Verification items for the finished model (mm, model axes). A direction names the side the tool comes from. Coordinates: 2 decimals unless noted, no trailing zeros. Write each loop counter-clockwise with the first axis right and the second up, starting at its lowest first coordinate (ties: lowest second). Pieces come first, ordered by that corner, then holes. Notation, with made-up numbers: (-20, 41.25) -> (25, 41.25) arc R23 cw to (25, 67.25) -> close; hole circle Ø4 at (37.25, -20). An arc over 180 degrees is marked (long way). Answer in a Markdown table with one row per item.
```python
from build123d import *

# Parameters (mm, degrees)
SKETCH1_W           = 15
SKETCH1_H           = 40
BOSS_EXTRUDE2_DEPTH = 3
SKETCH2_W           = 15
SKETCH2_H           = 15
BOSS_EXTRUDE5_DEPTH = 5
CUT_EXTRUDE9_DEPTH  = 15
SKETCH14_W          = 11
SKETCH14_H          = 0.5
CUT_EXTRUDE10_DEPTH = 5
BOSS_EXTRUDE9_DEPTH = 2
SKETCH18_R          = 1.5
CUT_EXTRUDE11_DEPTH = 10


with BuildPart() as part:
    # Sketch1 → Boss-Extrude2 (new body)
    with BuildSketch(Plane.XY):
        with Locations((0.416666667, -8.072916667)):
            Rectangle(SKETCH1_W, SKETCH1_H)
    extrude(amount=BOSS_EXTRUDE2_DEPTH)

    # Sketch2 → Boss-Extrude5 (add)
    with BuildSketch(Plane(origin=(0, 0, 0), x_dir=(-1, 0, 0), z_dir=(0, 0, -1))):
        with Locations((-0.416666667, 4.427083333)):
            Rectangle(SKETCH2_W, SKETCH2_H)
    extrude(amount=BOSS_EXTRUDE5_DEPTH)

    # Sketch12 → Cut-Extrude9 (cut)
    with BuildSketch(Plane.ZY.offset(7.083333333)):
        Polygon((-5, 11.927083333), (-5, 4.427083333), (0, 11.927083333), align=None)
    extrude(amount=-CUT_EXTRUDE9_DEPTH, mode=Mode.SUBTRACT)

    # Sketch14 → Cut-Extrude10 (cut)
    with BuildSketch(Plane(origin=(0, 3.669871795, -5.504807692), x_dir=(-1, 0, 0), z_dir=(0, 0.5547001962252293, -0.8320502943378436))):
        with Locations((-0.416666667, 3.160055009)):
            Rectangle(SKETCH14_W, SKETCH14_H)
        with Locations((-0.416666667, 4.160055009)):
            Rectangle(SKETCH14_W, SKETCH14_H)
        with Locations((-0.416666667, 5.160055009)):
            Rectangle(SKETCH14_W, SKETCH14_H)
        with Locations((-0.416666667, 6.160055009)):
            Rectangle(SKETCH14_W, SKETCH14_H)
        with Locations((-0.416666667, 7.160055009)):
            Rectangle(SKETCH14_W, SKETCH14_H)
    extrude(amount=-CUT_EXTRUDE10_DEPTH, mode=Mode.SUBTRACT)

    # Sketch17 → Boss-Extrude9 (add)
    with BuildSketch(Plane(origin=(0, -3.072916667, 0), x_dir=(-1, 0, 0), z_dir=(0, -1, 0))):
        with BuildLine():
            Line((-4.916666667, 4.5), (4.083333333, 4.5))
            ThreePointArc((4.083333333, 4.5), (6.083333333, 2.5), (4.083333333, 0.5))
            Line((4.083333333, 0.5), (-4.916666667, 0.5))
            ThreePointArc((-4.916666667, 0.5), (-6.916666667, 2.5), (-4.916666667, 4.5))
        make_face()
    extrude(amount=BOSS_EXTRUDE9_DEPTH)

    # Sketch18 → Cut-Extrude11 (cut)
    with BuildSketch(Plane.XZ.offset(5.072916667)):
        with Locations(Location((-4.083333333, -2.5, 0), (0, 0, 270))):
            Circle(SKETCH18_R)
        with Locations(Location((4.916666667, -2.5, 0), (0, 0, 270))):
            Circle(SKETCH18_R)
        with Locations(Location((0.416666667, -2.5, 0), (0, 0, 270))):
            Circle(SKETCH18_R)
    extrude(amount=-CUT_EXTRUDE11_DEPTH, mode=Mode.SUBTRACT)


solid = part.part
```
1. Mould release check, pull along Z, two halves, no side actions. Record for faces 5 (the flat face through (0.494, 5.34, -2.764)), 6 (the flat face through (7.917, -4, 1)), 7 (the flat face through (1, 1, -5)): released by +Z, released by -Z, zero draft, split by the parting line, or undercut.
Geometry says:
| item | result |
|---|---|
| face 5 | undercut |
| face 6 | zero draft |
| face 7 | released by -Z |
2. Section check C-C, the plane y = -15. Record the boundary of the cut face in (x, z), plus the area to 3 significant figures.
Geometry says:
| item | result |
|---|---|
| outline | (-7.08, 0) -> (7.92, 0) -> (7.92, 3) -> (-7.08, 3) -> close |
| area | 45.0 mm^2 |
3. Depth check by flat-ended pin: P1, Ø3.5, axis at x = 4.92, z = -2.5, coming from the +Y side; P2, Ø7.5, axis at x = -0.5, y = -18.5, coming from the -Z side; P3, Ø4, axis at x = 0.42, z = -2.5, coming from the +Y side. Enter the tip coordinate at first touch or a pass-through.
Geometry says:
| item | result |
|---|---|
| P1 | y = 10.8 |
| P2 | z = 0 |
| P3 | y = 11.18 |
4. Thickness scan on line 1 (X direction, y = 0.5, z = -2.5); line 2 (Z direction, x = 3.5, y = 6); line 3 (Y direction, x = -4.25, z = 1). Record the ranges inside material, lowest first. Write a range as from..to.
Geometry says:
| item | result |
|---|---|
| line 1 | -7.08..-5.58, -2.58..-1.08, 1.92..3.42, 6.42..7.92 |
| line 2 | -3.95..-3.75, -2.85..-1.95, -1.05..-0.15, 0.75..1.65, 2.06..3 |
| line 3 | -28.07..4.41, 4.63..5.23, 5.84..6.44, 7.04..7.64, 8.24..11.93 |
5. Tool access check on faces 1 (the flat face through (-5.083, 4.6, -1.2)), 2 (the flat face through (-4, 4.927, -3)), 3 (the cylindrical face through (6.916, -4.059, -2.456)), 4 (the flat face through (0, -4, -0.5)). Record the directions out of +Z, -Z, +X, -X, +Y, -Y that give a thin tool (end or side, any length) a straight path to the whole face; none if there is none.
Geometry says:
| item | result |
|---|---|
| face 1 | none |
| face 2 | -Y |
| face 3 | +X, -Y |
| face 4 | +X, -X, -Y |
6. Section check A-A, the plane y = -4.5. Record the boundary of the cut face in (x, z), plus the area to 3 significant figures.
Geometry says:
| item | result |
|---|---|
| outline | (-7.08, 0) -> (7.92, 0) -> (7.92, 3) -> (-7.08, 3) -> close; (-4.08, -4.5) -> (4.92, -4.5) arc R2 ccw to (4.92, -0.5) -> (-4.08, -0.5) arc R2 ccw to start; hole circle Ø3 at (-4.08, -2.5); hole circle Ø3 at (0.42, -2.5); hole circle Ø3 at (4.92, -2.5) |
| area | 72.4 mm^2 |
